Verification items for the finished model (mm, model axes). Face numbers are marked on the shaded views. A direction names the side the tool comes from. Round coordinates to 2 decimals unless told otherwise and drop trailing zeros. Order: outer loops, then holes, each group sorted by start corner. A loop starts at its lowest first (then second) coordinate and runs counter-clockwise, first axis right, second up. Notation, with made-up numbers: (-28, 54.5) -> (12, 54.5) arc R14 cw to (12, 74.5) -> close; hole circle Ø4 at (41, 21.25). An arc over 180 degrees is marked (long way). Return JSON: item names as keys, results as strings. Group by question number.
Item 1: Sectioned sample at D-D on x = -11.25. Record the cut outline in (y, z), plus the area to 3 significant figures.
Item 2: Depth check by flat-ended pin: pin 1 Ø3 at (x, z) = (-12, -2) entering from +Y; pin 2 Ø6 at (x, y) = (-3.5, 7) entering from -Z; pin 3 Ø1.3 at (y, z) = (-3.5, 9.5) entering from +X (3 decimals). Enter the tip coordinate at first touch or a pass-through.
Item 3: Access from +Z, -Z, +X, -X, +Y, -Y to the whole of each face (thin tool, end or side, straight path). Record for the marked faces 1, 2 and 3.
Item 4: Scan lines: probe 1 along Y at (x, z) = (-11.25, 9.5); probe 2 along Y at (x, z) = (-4, 5.25); probe 3 along X at (y, z) = (-2.4, 9.7) (3 decimals). Record each from-to range of solid material in increasing order. Write a range as from..to.
Item 5: Sectioned sample at C-C on y = -2.4. Record the cut outline in (x, z) (3 decimals), plus the area to 4 significant figures.
Item 6: Sectioned sample at B-B on y = 31.5. Record the cut outline in (x, z), plus the area to 4 significant figures.
Item 7: Sectioned sample at A-A on x = -18.5. Record the cut outline in (y, z).
```python
from build123d import *

# Parameters (mm, degrees)
SKETCH1_W               = 22.5
SKETCH1_H               = 37
SKETCH1_R               = 1.5
BOSS_EXTRUDE1_DEPTH     = 19
BOSS_EXTRUDE2_DEPTH     = 8
SKETCH2_W               = 5.15
SKETCH2_H               = 2.7
BOSS_EXTRUDE3_DEPTH     = 4.8
CUT_EXTRUDE1_DEPTH      = 47.217664372
CUT_EXTRUDE1_DEPTH_BACK = 47.217664372
SKETCH3_R               = 1.5


with BuildPart() as part:
    # Sketch1 → Boss-Extrude1 (new body)
    with BuildSketch(Plane.XY):
        with Locations((-11.25, 18.5)):
            Rectangle(SKETCH1_W, SKETCH1_H)
        with Locations((-4, 31.5)):
            Circle(SKETCH1_R, mode=Mode.SUBTRACT)
        with Locations((-18.5, 31.5)):
            Circle(SKETCH1_R, mode=Mode.SUBTRACT)
    extrude(amount=BOSS_EXTRUDE1_DEPTH)

    # Sketch1_3 → Boss-Extrude2 (add)
    with BuildSketch(Plane.XY):
        with BuildLine():
            ThreePointArc((-9.418482828, 12.4), (-8.6, 10.55), (-9.418482828, 8.7))
            Line((-9.418482828, 8.7), (-13.081517172, 8.7))
            ThreePointArc((-13.081517172, 8.7), (-13.9, 10.55), (-13.081517172, 12.4))
            Line((-13.081517172, 12.4), (-9.418482828, 12.4))
        make_face()
    extrude(amount=-BOSS_EXTRUDE2_DEPTH)

    # Sketch2 → Boss-Extrude3 (add)
    with BuildSketch(Plane.XZ):
        with Locations((-11.25, 9.5)):
            Rectangle(SKETCH2_W, SKETCH2_H)
    extrude(amount=BOSS_EXTRUDE3_DEPTH)

    # Sketch3 → Cut-Extrude1 (cut, two sides: drawn at the far end of the back side and taken through both)
    with BuildSketch(Plane(origin=(0, 0, 8.15), x_dir=(-1, 0, 0), z_dir=(0, 0, -1)).offset(-CUT_EXTRUDE1_DEPTH_BACK)):
        with Locations((11.25, -2.4)):
            Circle(SKETCH3_R)
    extrude(amount=CUT_EXTRUDE1_DEPTH + CUT_EXTRUDE1_DEPTH_BACK, mode=Mode.SUBTRACT)


solid = part.part
```
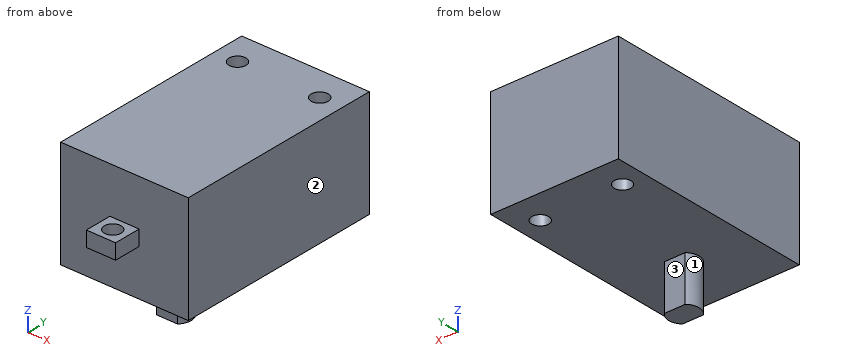
Recorded:
{
 "1": {"outline": "(-4.8, 8.15) -> (-3.9, 8.15) -> (-3.9, 10.85) -> (-4.8, 10.85) -> close; (-0.9, 8.15) -> (0, 8.15) -> (0, 0) -> (8.7, 0) -> (8.7, -8) -> (12.4, -8) -> (12.4, 0) -> (37, 0) -> (37, 19) -> (0, 19) -> (0, 10.85) -> (-0.9, 10.85) -> close", "area": "737 mm²"},
 "2": {"pin 1": "y = 12.4", "pin 2": "z = 0", "pin 3": "x = -8.675"},
 "3": {"face 1": "-Z, -X", "face 2": "+Z, -Z, +X, +Y, -Y", "face 3": "-Z, +X, -X, +Y"},
 "4": {"probe 1": "-4.8..-3.9, -0.9..37", "probe 2": "0..30, 33..37", "probe 3": "-13.825..-12.75, -9.75..-8.675"},
 "5": {"outline": "(-13.825, 8.15) -> (-12.75, 8.15) -> (-12.75, 10.85) -> (-13.825, 10.85) -> close; (-9.75, 8.15) -> (-8.675, 8.15) -> (-8.675, 10.85) -> (-9.75, 10.85) -> close", "area": "5.805 mm²"},
 "6": {"outline": "(-22.5, 0) -> (-20, 0) -> (-20, 19) -> (-22.5, 19) -> close; (-17, 0) -> (-5.5, 0) -> (-5.5, 19) -> (-17, 19) -> close; (-2.5, 0) -> (0, 0) -> (0, 19) -> (-2.5, 19) -> close", "area": "313.5 mm²"},
 "7": {"outline": "(0, 0) -> (30, 0) -> (30, 19) -> (0, 19) -> close; (33, 0) -> (37, 0) -> (37, 19) -> (33, 19) -> close"}
}
